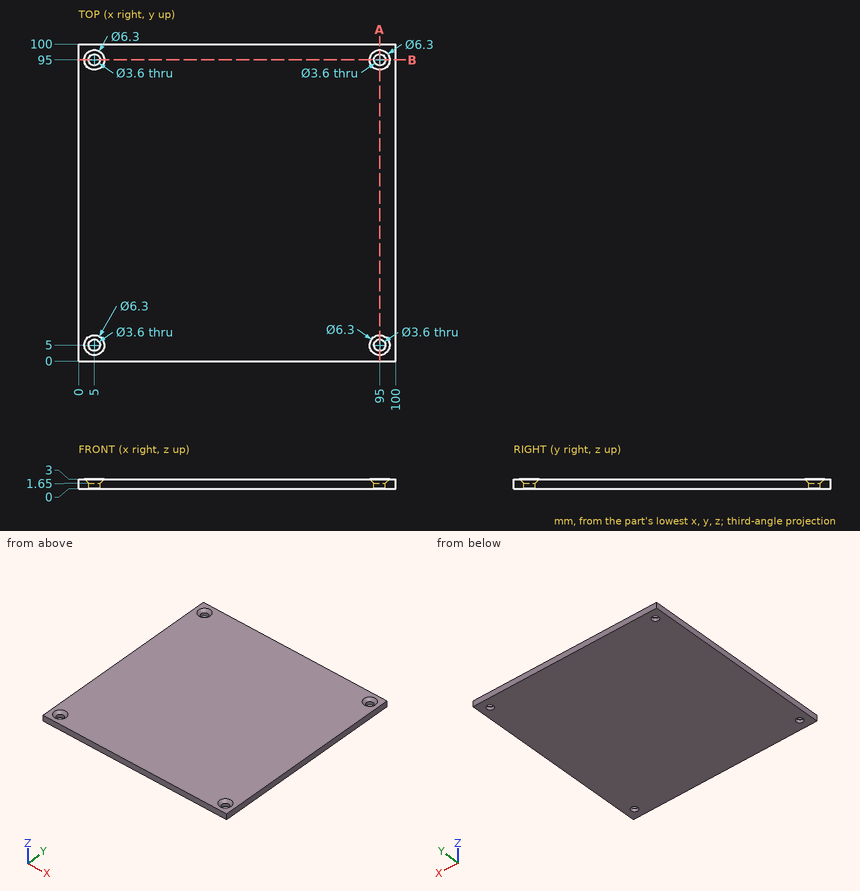
The figure shows three views and two pictorial views of one solid part (mm, origin at its lowest corner). Answer the questions. Give positions to 0.01 mm unless a question says otherwise; leave off trailing zeros. Write each loop counter-clockwise with the first axis right and the second up, starting at its lowest first coordinate (ties: lowest second). Pieces come first, ordered by that corner, then holes. Notation, with made-up numbers: M 38.25,-38 L 77.25,-38 A8 cw 77.25,-30 Z; hole C -6,29 d9. An arc over 180 degrees is marked long. One line per item, written item: value. Start each with the question number.
(1) Find section A-A (x = 95). Determine the outline of the cut face in (y, z), plus the area to 3 significant figures.
(2) Find the intervals of material crossed by line 1 (X direction, y = 95, z = 0.55); line 2 (Y direction, x = 94, z = 2.25), in increasing order.
(3) Flat-ended cylindrical pins translate along their axes: pin 1 Ø4.5 at (x, y) = (5, 95) entering from +Z; pin 2 Ø6 at (x, y) = (5, 5) entering from +Z. Find the tip coordinate at first contact, or state that the pin passes through.
Results below:
1. outline: M 0,0 L 3.2,0 L 3.2,1.65 L 1.85,3 L 0,3 Z; M 6.8,0 L 93.2,0 L 93.2,1.65 L 91.85,3 L 8.15,3 L 6.8,1.65 Z; M 96.8,0 L 100,0 L 100,3 L 98.15,3 L 96.8,1.65 Z
1. area: 275 mm^2
2. line 1: x = 0 to 3.2, 6.8 to 93.2, 96.8 to 100
2. line 2: y = 0 to 2.82, 7.18 to 92.82, 97.18 to 100
3. pin 1: stops at z = 2.1
3. pin 2: stops at z = 2.85
